Autodesk Inventor part; units mm, degrees
ref_plane "YZ Plane" through (0, 0, 0) normal (1, 0, 0) x (0, 1, 0)
ref_plane "XZ Plane" through (0, 0, 0) normal (0, 1, 0) x (-1, 0, 0)
ref_plane "XY Plane" through (0, 0, 0) normal (0, 0, 1) x (1, 0, 0)
sketch "Sketch1" plane through (0, 0, 0) normal (0, 0, 1) x (1, 0, 0)
  line L0 (0, 0) -> (12.7, 0)
  line L1 (14.7, 0) -> (14.7, 3.5) construction
  line L2 (14.7, 3.5) -> (12.7, 3.5) construction
  line L3 (0, 0) -> (0, 2)
  line L4 (12.7, 3.5) -> (12.7, 4) construction
  line L5 (14.7, 3.5) -> (12.7, 4)
  line L6 (14.7, 3.5) -> (12.7, 0)
  line L7 (12.7, 4) -> (11.5571, 2)
  line L8 (0, 2) -> (11.5571, 2)
  dimension "d0" = 14.7
  dimension "d1" = 3.5
  dimension "d2" = 2
  dimension "d3" = 0.5
  dimension "d4" = 2
  dimension "d10" = 2
revolve "Revolution1" add sketch "Sketch1" angle 360 about axis through (0, 0, 0) along (0, 1, 0)
sketch "Sketch2" plane through (0, 2, 0) normal (0, 1, 0) x (1, 0, 0)
  circle A0 centre (0, 0) radius 4.7
  dimension "d6" = 9.4
extrude "Extrusion1" cut sketch "Sketch2" against normal through all
fillet "Fillet1" radius 3 1 edges at (-12.7, 0, 0)
properties part number "BottomBushingWasher" material "Aluminum"
Work out the finished part from the listing and answer in its coordinate system (mm). A direction names the side the tool comes from. Round coordinates to 2 decimals unless told otherwise and drop trailing zeros. Write each loop counter-clockwise with the first axis right and the second up, starting at its lowest first coordinate (ties: lowest second). Pieces come first, ordered by that corner, then holes.
1) A cutting plane is placed at C-C on y = 2.6. Determine the outline of the cut face in (x, z), and give its area (3 significant figures).
2) Flat-ended cylindrical pins translate along their axes: P1, Ø4, axis at x = -3, z = 11, coming from the +Y side; P2, Ø11.5, axis at x = -0.5, z = -5, coming from the +Y side. Find the tip coordinate at first contact, or state that the pin passes through.
3) Consider probe 1 along Z at (x, y) = (0, 1.5); probe 2 along Y at (x, z) = (-7.75, 7); probe 3 along Z at (x, y) = (0, 3.2). Determine where each line is inside the solid, lowest interval first.
4) A cutting plane is placed at A-A on x = 0. Determine the outline of the cut face in (y, z), and give its area (3 significant figures).
5) A cutting plane is placed at B-B on z = 0. Determine the outline of the cut face in (x, y), and give its area (3 significant figures).
6) Determine the mould class of faces 1 (the face through (-9.23, 2.13, 7.08)), 2 (the face through (5, 0, 0)) for opening direction Z: pulls with the +Z half, pulls with the -Z half, needs draft (parallel to the pull), parting line crosses it, or undercut.
7) Which of the six approach directions +Z, -Z, +X, -X, +Y, -Y give full straight-line access (tool end or side, diameter ignored) to faces 3 (the face through (-1.02, 1.01, 4.59)), 4 (the face through (0, 2, 5))?
Entries:
1. outline: circle Ø28.37 at (0, 0); hole circle Ø23.8 at (0, 0)
1. area: 187 mm2
2. P1: stops at y = 4
2. P2: stops at y = 2
3. probe 1: z = -13.56 to -4.7, 4.7 to 13.56
3. probe 2: y = 0 to 2
3. probe 3: z = -14.53 to -12.24, 12.24 to 14.53
4. outline: (0, -10.96) arc R3 ccw to (1.51, -13.56) - (3.5, -14.7) - (4, -12.7) - (2, -11.56) - (2, -4.7) - (0, -4.7) - close; (0, 4.7) - (2, 4.7) - (2, 11.56) - (4, 12.7) - (3.5, 14.7) - (1.51, 13.56) arc R3 ccw to (0, 10.96) - close
4. area: 41.3 mm2
5. outline: (-14.7, 3.5) - (-13.56, 1.51) arc R3 ccw to (-10.96, 0) - (-4.7, 0) - (-4.7, 2) - (-11.56, 2) - (-12.7, 4) - close; (4.7, 0) - (10.96, 0) arc R3 ccw to (13.56, 1.51) - (14.7, 3.5) - (12.7, 4) - (11.56, 2) - (4.7, 2) - close
5. area: 41.3 mm2
6. face 1: undercut
6. face 2: needs draft
7. face 3: +Y, -Y
7. face 4: +Y
